Autodesk Fusion 360 part; units mm, degrees
sketch "Sketch1" plane through (0, 0, 0) normal (0, 1, 0) x (1, 0, 0)
  circle A0 centre (0, 0) radius 38.1
  dimension "d1" = 76.2
extrude "Extrude1" add sketch "Sketch1" against normal blind 6.35
sketch "Sketch2" plane through (0, -6.35, 0) normal (0, -1, 0) x (1, 0, 0)
  circle A0 centre (0, 0) radius 38.1
  circle A1 centre (0, 0) radius 15.875
  dimension "d4" = 31.75
extrude "Extrude2" cut sketch "Sketch2" against normal blind 83.82 contours A1
sketch "Sketch3" plane through (0, -6.35, 0) normal (0, -1, 0) x (1, 0, 0)
  circle A0 centre (0, 0) radius 15.875
  circle A1 centre (0, 0) radius 38.1
  circle A2 centre (0, 0) radius 15.875
  circle A3 centre (0, 0) radius 19.05
  dimension "d7" = 31.75
  dimension "d8" = 38.1
extrude "Extrude3" add sketch "Sketch3" along normal blind 50.8 contours A3
fillet "Fillet1" radius 2.54 1 edges at (-17.7608, -6.35, 6.8888)
sketch "Sketch4" plane through (0, 0, 0) normal (0, 1, 0) x (-1, 0, 0)
  circle A0 centre (0, 0) radius 15.875
  circle A1 centre (0, 0) radius 38.1
  circle A2 centre (0, 26.9875) radius 3.175
  circle A3 centre (-19.083, 19.083) radius 3.175
  circle A4 centre (-26.9875, 0) radius 3.175
  circle A5 centre (-19.083, -19.083) radius 3.175
  circle A6 centre (0, -26.9875) radius 3.175
  circle A7 centre (19.083, -19.083) radius 3.175
  circle A8 centre (26.9875, 0) radius 3.175
  circle A9 centre (19.083, 19.083) radius 3.175
  dimension "d13" = 6.35
  dimension "d15" = 360
extrude "Extrude4" cut sketch "Sketch4" against normal blind 76.2 contours A2 | A3 | A4 | A5 | A6 | A7 | A8 | A9
sketch "Sketch5" plane through (0, 0, 0) normal (0, 1, 0) x (-1, 0, 0)
  circle A0 centre (0, 26.9875) radius 3.175
  circle A1 centre (0, -26.9875) radius 3.175
  circle A2 centre (19.083, -19.083) radius 3.175
  circle A3 centre (-19.083, 19.083) radius 3.175
  circle A4 centre (19.083, 19.083) radius 3.175
  circle A5 centre (-19.083, -19.083) radius 3.175
  circle A6 centre (26.9875, 0) radius 3.175
  circle A7 centre (-26.9875, 0) radius 3.175
  circle A8 centre (0, 0) radius 15.875
  circle A9 centre (0, 0) radius 38.1
  line L0 (-2.54, 15.875) -> (-2.54, -15.875)
  line L1 (2.54, 15.875) -> (2.54, -15.875)
  arc A10 (-2.54, -15.6705) -> (2.54, -15.6705) centre (0, 0) ccw
  arc A11 (2.54, 15.6705) -> (-2.54, 15.6705) centre (0, 0) ccw
extrude "Extrude5" add sketch "Sketch5" against normal blind 12.7 contours A8 L0 L1 A10 A11
The listing builds one solid part. Answer for the finished solid, in the listing's coordinates (mm). A direction names the side the tool comes from. Coordinates: 2 decimals unless noted, no trailing zeros. Write each loop counter-clockwise with the first axis right and the second up, starting at its lowest first coordinate (ties: lowest second). Pieces come first, ordered by that corner, then holes. Notation, with made-up numbers: M -7.5,2.5 L 15.5,2.5 A17 cw 15.5,9.5 Z; hole C 5.25,41.25 d4. An arc over 180 degrees is marked long. Put each result on its own line as item: value. Start each with the question number.
1. Flat-ended cylindrical pins translate along their axes: P1, Ø8, axis at x = 22.5, z = 17.5, coming from the -Y side; P2, Ø3, axis at y = -46, z = 15.5, coming from the -X side; P3, Ø12, axis at x = -7.5, y = -34.5, coming from the +Z side. Find the tip coordinate at first contact, or state that the pin passes through.
2. Which of the six approach directions +Z, -Z, +X, -X, +Y, -Y give full straight-line access (tool end or side, diameter ignored) to faces 1 (the flat face through (2.54, -6, 0)), 2 (the flat face through (16, -6.35, 16)), 3 (the flat face through (1, 0, 1))?
3. A cutting plane is placed at A-A on z = 0. Count the separate pieces of the cut face and the enclosed holes in it, then the cut area to 3 significant figures.
4. Consider line 1 (X direction, y = -10, z = -6); line 2 (Y direction, x = -23.5, z = -24.5); line 3 (X direction, y = -40.5, z = -10). Determine where each line is inside the solid, lowest interval first. Write a range as from..to.
5. A cutting plane is placed at C-C on z = -28.5. Write down the section's boundary in (x, y), then the cut area to 3 significant figures.
6. A cutting plane is placed at D-D on x = 25.5. Write down the section's boundary in (y, z), then the cut area to 3 significant figures.
7. For a pull along X with two mould halves and no side action, classify faces 4 (the flat face through (-4, -57.15, 16)), 5 (the cylindrical face through (-30.235, -3.131, 23.183)), 6 (the cylindrical face through (16.055, -3.131, 20.037)), 7 (the cylindrical face through (16.055, -3.131, -18.129)) as pulls with the +X half, pulls with the -X half, needs draft (parallel to the pull), parting line crosses it, or undercut.
Resolved:
1. P1: stops at y = -6.35
1. P2: stops at x = -12.92
1. P3: stops at z = 18.99
2. face 1: +Y, -Y
2. face 2: -Y
2. face 3: +Z, -Z, +X, -X, +Y
3. separate pieces: 5
3. enclosed holes: 0
3. area: 591 mm2
4. line 1: x = -18.08..-14.7, -2.54..2.54, 14.7..18.08
4. line 2: y = -6.35..0
4. line 3: x = -16.21..-12.33, 12.33..16.21
5. outline: M -25.29,-6.35 L -2.79,-6.35 L -2.79,0 L -25.29,0 Z; M 2.79,-6.35 L 25.29,-6.35 L 25.29,0 L 2.79,0 Z
5. area: 286 mm2
6. outline: M -6.35,-28.31 L 0,-28.31 L 0,-2.8 L -6.35,-2.8 Z; M -6.35,2.8 L 0,2.8 L 0,28.31 L -6.35,28.31 Z
6. area: 324 mm2
7. face 4: needs draft
7. face 5: parting line crosses it
7. face 6: undercut
7. face 7: undercut
